from build123d import *

# Parameters (mm, degrees)
PAD_DEPTH    = 78
SKETCH001_R  = 1.25
POCKET_DEPTH = 5
CHAMFER_SIZE = 1.5


with BuildPart() as part:
    # Sketch → Pad (new body)
    with BuildSketch(Plane.YZ):
        Polygon((0, 0), (25, 0), (25, 1.5), (23, 3.2), (2, 3.2), (0, 1.5), align=None)
    extrude(amount=PAD_DEPTH)

    # Sketch001 (on Face4 of Pad) → Pocket (cut)
    with BuildSketch(Plane(origin=(0, 0, 3.2), x_dir=(0, -1, 0), z_dir=(0, 0, 1))):
        with Locations((-12.75, 3)):
            Circle(SKETCH001_R)
    extrude(amount=-POCKET_DEPTH, mode=Mode.SUBTRACT)

    # Chamfer
    chamfer_edges = [part.edges().sort_by_distance(p)[0] for p in [
        (3, 14, 3.2),
    ]]
    chamfer(chamfer_edges, length=CHAMFER_SIZE)


solid = part.part
Work out the finished part from the listing and answer in its coordinate system (mm). Coordinates: 2 decimals unless noted, no trailing zeros. Write each loop counter-clockwise with the first axis right and the second up, starting at its lowest first coordinate (ties: lowest second). Pieces come first, ordered by that corner, then holes. Notation, with made-up numbers: (14, 16.5) - (51, 16.5) arc R26 ccw to (51, 42.5) - close; hole circle Ø9 at (78, -23.5). An arc over 180 degrees is marked (long way). One line per question, with ' | ' between items.
1) Consider probe 1 along X at (y, z) = (12.75, 0.5); probe 2 along X at (y, z) = (13.5, 0.5); probe 3 along Y at (x, z) = (4, 2.9). Determine where each line is inside the solid, lowest interval first. Write a range as [from, to].
Checks:
probe 1: [0, 1.75], [4.25, 78] | probe 2: [0, 2], [4, 78] | probe 3: [1.65, 10.51], [14.99, 23.35]
2) Find section A-A, the plane x = 3. Determine the outline of the cut face in (y, z).
Checks:
outline: (0, 0) - (11.5, 0) - (11.5, 1.7) - (10, 3.2) - (2, 3.2) - (0, 1.5) - close; (14, 0) - (25, 0) - (25, 1.5) - (23, 3.2) - (15.5, 3.2) - (14, 1.7) - close
3) Find section C-C, the plane x = 22.5. Determine the outline of the cut face in (y, z).
Checks:
outline: (0, 0) - (25, 0) - (25, 1.5) - (23, 3.2) - (2, 3.2) - (0, 1.5) - close
4) A flat-ended cylindrical pin translates along its axis: P1, Ø8, axis at x = 17.5, y = 3, coming from the -Z side. Find the tip coordinate at first contact, or state that the pin passes through.
Checks:
P1: z = 0
5) Find section B-B, the plane y = 12.75. Determine the outline of the cut face in (x, z), and give its area (3 significant figures).
Checks:
outline: (0, 0) - (1.75, 0) - (1.75, 1.7) - (0.25, 3.2) - (0, 3.2) - close; (4.25, 0) - (78, 0) - (78, 3.2) - (5.75, 3.2) - (4.25, 1.7) - close | area: 239 mm2
6) The mould has two halves that part along X. Classify faces 1 (the face through (3.845, 13.671, 0.862)), 2 (the face through (0, 12, 2)), 3 (the face through (38.45, 24.01, 2.34)): +X half, -X half, draft (parallel to the pull), parting line (faces both ways), or undercut.
Checks:
face 1: undercut | face 2: -X half | face 3: draft
